```python
from build123d import *

# Parameters (mm, degrees)
EXTRUDE_1_DEPTH     = 10
SKETCH_2_R          = 8.2
CUT_EXTRUDE_1_DEPTH = 10
SKETCH_3_R          = 7.8
EXTRUDE_2_DEPTH     = 2
CUT_EXTRUDE_2_DEPTH = 244.001178821
CHAMFER_1_SIZE      = 2
SKETCH_12_R         = 12.2
CUT_EXTRUDE_3_DEPTH = 2


with BuildPart() as part:
    # 草图1 → 凸台-拉伸1 (new body)
    with BuildSketch(Plane(origin=(0, 0, 0), x_dir=(1, 0, 0), z_dir=(0, 1, 0))):
        with BuildLine():
            ThreePointArc((38.135472776, -1.298351331), (42.500736357, 11.388037985), (32.377112543, 20.192141624))
            Line((32.377112543, 20.192141624), (2.934972204, 23.819864361))
            ThreePointArc((2.934972204, 23.819864361), (2.523648479, 23.866947822), (2.111573774, 23.906929042))
            add(Edge.make_bspline(
                [(2.111573774, 23.906929042), (-9.810921984, 24.95998062), (-117.579356421, 40.552472419), (-200.501701748, 36.233495272), (-230.78473121, 16.843086794)],
                knots=[0, 0, 0, 0, 0.545538067, 1, 1, 1, 1], degree=3))
            ThreePointArc((-230.78473121, 16.843086794), (-233.515274748, -14.74236577), (-202.285423784, -9.284061046))
            add(Edge.make_bspline(
                [(-16.047074382, -17.846327459), (-50.225325952, 12.886098942), (-142.28144772, 36.786073578), (-197.939957095, -0.992635508), (-202.285423784, -9.284061046)],
                knots=[0, 0, 0, 0, 0.861614938, 1, 1, 1, 1], degree=3))
            ThreePointArc((-16.047074382, -17.846327459), (-8.21278774, -22.551055797), (0.812217897, -23.986252356))
            ThreePointArc((0.812217897, -23.986252356), (8.004199727, -22.625931732), (14.451692669, -19.161121549))
            Line((14.451692669, -19.161121549), (38.135472776, -1.298351331))
        make_face()
    extrude(amount=EXTRUDE_1_DEPTH)

    # 草图2 → 切除-拉伸1 (cut)
    with BuildSketch(Plane(origin=(0, 10, 0), x_dir=(1, 0, 0), z_dir=(0, 1, 0))):
        with Locations(Location((0, 0, 0), (0, 0, 270))):
            Circle(SKETCH_2_R)
    extrude(amount=-CUT_EXTRUDE_1_DEPTH, mode=Mode.SUBTRACT)

    # 草图3 → 凸台-拉伸2 (add)
    with BuildSketch(Plane(origin=(0, 10, 0), x_dir=(1, 0, 0), z_dir=(0, 1, 0))):
        with Locations(Location((30.909626441, 8.282209443, 0), (0, 0, 270))):
            Circle(SKETCH_3_R)
    extrude(amount=EXTRUDE_2_DEPTH)

    # 草图6 → 切除-拉伸2 (cut, through all)
    with BuildSketch(Plane(origin=(0, 10, 0), x_dir=(1, 0, 0), z_dir=(0, 1, 0))):
        Polygon((-208.452994616, 0), (-214.226497308, 10), (-225.773502692, 10), (-231.547005384, 0), (-225.773502692, -10), (-214.226497308, -10), align=None)
    extrude(amount=-CUT_EXTRUDE_2_DEPTH, mode=Mode.SUBTRACT)

    # 倒角1
    chamfer_1_edges = [part.edges().sort_by_distance(p)[0] for p in [
        (-109.293214932, 0, -18.683029708),
        (2.523648479, 0, -23.866947822),
        (-233.515274748, 0, 14.74236577),
        (17.656042374, 0, -22.006002992),
        (-109.293214932, 0, -18.683029708),
        (42.500736357, 0, -11.388037985),
        (-1.033673825, 0, 23.977729634),
        (26.293582722, 0, 10.22973644),
        (-109.293214932, 10, -18.683029708),
        (2.523648479, 10, -23.866947822),
        (-233.515274748, 10, 14.74236577),
        (17.656042374, 10, -22.006002992),
        (-109.293214932, 10, -18.683029708),
        (42.500736357, 10, -11.388037985),
        (-1.033673825, 10, 23.977729634),
        (26.293582722, 10, 10.22973644),
    ]]
    chamfer(chamfer_1_edges, length=CHAMFER_1_SIZE)

    # 草图12 → 切除-拉伸3 (cut)
    with BuildSketch(Plane(origin=(0, 10, 0), x_dir=(1, 0, 0), z_dir=(0, 1, 0))):
        with Locations(Location((0, 0, 0), (0, 0, 270))):
            Circle(SKETCH_12_R)
    extrude(amount=-CUT_EXTRUDE_3_DEPTH, mode=Mode.SUBTRACT)


solid = part.part
```
Part model, mm, in its own coordinate system. A direction names the side the tool comes from. Round coordinates to 2 decimals unless told otherwise and drop trailing zeros.
Item 1: Drill centre lines: line 1 (X direction, y = 9.45, z = 0); line 2 (X direction, y = 1.75, z = -3) (3 decimals); line 3 (X direction, y = 6.5, z = 14.5). Where is each one in solid material? Low to high.
Item 2: 3-axis set-ups, long thin cutter, end or side, ignore diameter. For faces 4 (the face through (-211.38, 5.07, 5.07)), 5 (the face through (42.55, 4.96, -11.2)), 6 (the face through (37.487, 10.986, -4.089)): which of +Z, -Z, +X, -X, +Y, -Y reach the whole face in a straight line?
Item 3: Cut at A-A, the plane z = 4. State how many separate pieces and enclosed holes the cut face has, then the cut area to 3 significant figures.
Item 4: Drop flat-ended pins along their axis: P1, Ø2, axis at x = -56.5, y = 8.5, coming from the -Z side; P2, Ø5, axis at y = 3, z = 1, coming from the -X side; P3, Ø21.5, axis at x = 0, z = 0, coming from the +Y side; P4, Ø4, axis at y = 8.5, z = -19, coming from the -X side. Give the stop position or say it passes through.
Item 5: Mould opens along Z. For faces 1 (the face through (25.866, 1.014, 9.317)), 2 (the face through (-231.902, 0.125, 13.67)), 3 (the face through (-7.4, 9, -9.7)) say: +Z half, -Z half, draft (parallel to the pull), parting line (faces both ways), or undercut.
A:
1. line 1: x = -238.55 to -231.55, -208.45 to -197.02, -39.99 to -12.2, 12.2 to 37.44
1. line 2: x = -239.521 to -229.815, -210.185 to -191.477, -48.975 to -7.632, 7.632 to 41.405
1. line 3: x = -233.77 to -206.23, -20 to 20.63
2. face 4: +Y, -Y
2. face 5: +X, +Y, -Y
2. face 6: +Y
3. separate pieces: 4
3. enclosed holes: 0
3. area: 741 mm2
4. P1: stops at z = -30.87
4. P2: stops at x = -240
4. P3: stops at y = 8
4. P4: stops at x = -230.44
5. face 1: +Z half
5. face 2: parting line
5. face 3: undercut
